from build123d import *

# Parameters (mm, degrees)
SKETCH2_R   = 4.7625
SKETCH2_R_2 = 3.8735


with BuildPart() as part:
    # Sweep1: sweep along a path in Sketch1
    with BuildLine(Plane.XY) as sweep1_path:
        Line((0, -127), (0, -23.8125))
        ThreePointArc((0, -23.8125), (6.974519773, -6.974519773), (23.8125, 0))
        Line((23.8125, 0), (38.1, 0))
    # Sketch2 → Sweep1 (sweep)
    with BuildSketch(Plane(origin=(38.1, 0, 0), x_dir=(0, 0, -1), z_dir=(1, 0, 0))):
        Circle(SKETCH2_R)
        Circle(SKETCH2_R_2, mode=Mode.SUBTRACT)
    sweep(path=sweep1_path.line)


solid = part.part
Can you work these out from the model? Positions are in its coordinate system, mm. A direction names the side the tool comes from. Round coordinates to 2 decimals unless told otherwise and drop trailing zeros. Loops run counter-clockwise (first coordinate to the right, second up) from the corner with the lowest first, then second, coordinate; pieces in that order, holes last. Notation, with made-up numbers: (32, -10.75) - (44, -10.75) arc R22 ccw to (44, 24.25) - close; hole circle Ø11 at (50, 27). An arc over 180 degrees is marked (long way). Use CSV: the item, a comma, the result in double quotes. Start each with the question number.
1) For pin 1 Ø4 at (y, z) = (-64.5, 3) entering from -X; pin 2 Ø2 at (y, z) = (-14.5, 3.5) entering from +X; pin 3 Ø4 at (y, z) = (-23, -0.5) entering from +X, each with a flat end and sliding along its axis, tell me the tip position at first contact or that it passes through.
2) We'd pull the mould along Z, two halves only. Please class faces 3 (the cylindrical face through (2.9, -74.68, 3.78)), 4 (the flat face through (-4, -127, 1)), 5 (the cylindrical face through (31.06, 3.27, -2.08)), 6 (the cylindrical face through (-3.27, -74.68, -2.08)): released by +Z, released by -Z, zero draft, split by the parting line, or undercut.
3) Please list where this line runs through material, in increasing order: probe 1 along Z at (x, y) = (29, 0). Write a range as [from, to].
4) If we section it at B-B on x = 28: Write out the boundary of the cut face in (y, z) (1 decimal), plus the area to 3 significant figures.
5) For faces 1 (the flat face through (38.1, 4, 1)), 2 (the cylindrical face through (31.06, -2.9, 3.78)), which set-ups out of +Z, -Z, +X, -X, +Y, -Y let a thin tool reach every point of the face, with its end or its side?
Geometry results:
1,pin 1,"stops at x = -4.66"
1,pin 2,"stops at x = 6.57"
1,pin 3,"stops at x = 4.96"
2,face 3,"split by the parting line"
2,face 4,"zero draft"
2,face 5,"undercut"
2,face 6,"undercut"
3,probe 1,"z = [-4.76, -3.87], [3.87, 4.76]"
4,outline,"circle Ø9.5 at (0, 0); hole circle Ø7.7 at (0, 0)"
4,area,"24.1 mm2"
5,face 1,"+Z, -Z, +X, +Y, -Y"
5,face 2,"+X"
